Check sheet for the modelled part. Datum: model origin and axes. Units: mm. A direction names the side the tool comes from. Round coordinates to 2 decimals unless told otherwise and drop trailing zeros. Write each loop counter-clockwise with the first axis right and the second up, starting at its lowest first coordinate (ties: lowest second). Pieces come first, ordered by that corner, then holes.
from build123d import *

# Parameters (mm, degrees)
BOSS_EXTRU_1_DEPTH      = 18.275
ESQUISSE2_W             = 40
ESQUISSE2_H             = 22
BOSS_EXTRU_2_DEPTH      = 3
ESQUISSE3_W             = 40
ESQUISSE3_H             = 2
BOSS_EXTRU_3_DEPTH      = 2
ESQUISSE4_W             = 20
ESQUISSE4_H             = 2
ENL_V_MAT_EXTRU_2_DEPTH = 22.275
ENL_V_START             = -7.775
ESQUISSE5_W             = 31.2
ESQUISSE5_H             = 5
ENL_V_MAT_EXTRU_3_DEPTH = 7.775
ESQUISSE6_W             = 34
ESQUISSE6_H             = 5.725
ENL_V_MAT_EXTRU_4_DEPTH = 12.5
BOSS_EXTRU_4_DEPTH      = 21.275
ESQUISSE8_W             = 34
ESQUISSE8_H             = 5.725
ENL_V_MAT_EXTRU_5_DEPTH = 11.946457824


with BuildPart() as part:
    # Esquisse1 → Boss.-Extru.1 (new body)
    with BuildSketch(Plane.XY):
        Polygon((-15.6, -80), (-20, -80), (-20, -60), (20, -60), (20, -80), (15.6, -80), (15.6, -76.5), (8.8, -76.5), (8.8, -71.5), (-8.8, -71.5), (-8.8, -76.5), (-15.6, -76.5), align=None)
    extrude(amount=BOSS_EXTRU_1_DEPTH)

    # Esquisse2 → Boss.-Extru.2 (add)
    with BuildSketch(Plane.XY.offset(18.275)):
        with Locations((0, -71)):
            Rectangle(ESQUISSE2_W, ESQUISSE2_H)
    extrude(amount=BOSS_EXTRU_2_DEPTH)

    # Esquisse3 → Boss.-Extru.3 (add)
    with BuildSketch(Plane(origin=(0, 0, 18.275), x_dir=(-1, 0, 0), z_dir=(0, 0, -1))):
        with Locations((0, -81)):
            Rectangle(ESQUISSE3_W, ESQUISSE3_H)
    extrude(amount=BOSS_EXTRU_3_DEPTH)

    # Esquisse4 → Enlèv. mat.-Extru.2 (cut, through all)
    with BuildSketch(Plane.XY.offset(21.275)):
        with Locations((0, -81)):
            Rectangle(ESQUISSE4_W, ESQUISSE4_H)
    extrude(amount=-ENL_V_MAT_EXTRU_2_DEPTH, mode=Mode.SUBTRACT)

    # Esquisse5 → Enlèv. mat.-Extru.3 (cut)
    with BuildSketch(Plane(origin=(0, 0, 0), x_dir=(-1, 0, 0), z_dir=(0, 0, -1)).offset(ENL_V_START)):
        with Locations((0, -74)):
            Rectangle(ESQUISSE5_W, ESQUISSE5_H)
    extrude(amount=ENL_V_MAT_EXTRU_3_DEPTH, mode=Mode.SUBTRACT)

    # Esquisse6 → Enlèv. mat.-Extru.4 (cut, through all)
    with BuildSketch(Plane.XZ.offset(71.5)):
        with Locations((0, 2.8625)):
            Rectangle(ESQUISSE6_W, ESQUISSE6_H)
    extrude(amount=-ENL_V_MAT_EXTRU_4_DEPTH, mode=Mode.SUBTRACT)

    # Esquisse7 → Boss.-Extru.4 (add)
    with BuildSketch(Plane.XY.offset(21.275)):
        with BuildLine():
            Line((-30, -49.053542176), (-20, -82))
            Line((-20, -82), (-18, -82))
            Line((-18, -82), (-18, -60))
            Line((-18, -60), (18, -60))
            Line((18, -60), (18, -82))
            Line((18, -82), (20, -82))
            Line((20, -82), (30, -49.053542176))
            ThreePointArc((30, -49.053542176), (0, -57.5), (-30, -49.053542176))
        make_face()
    extrude(amount=-BOSS_EXTRU_4_DEPTH)

    # Esquisse8 → Enlèv. mat.-Extru.5 (cut, through all)
    with BuildSketch(Plane.XZ.offset(60)):
        with Locations((0, 2.8625)):
            Rectangle(ESQUISSE8_W, ESQUISSE8_H)
    extrude(amount=-ENL_V_MAT_EXTRU_5_DEPTH, mode=Mode.SUBTRACT)


solid = part.part
1. Sectioned sample at D-D, the plane y = -65. Enter the section's corners in (x, z) (3 decimals), plus the area to 3 significant figures.
2. Sectioned sample at B-B, the plane z = 11.25. Enter the section's corners in (x, y), plus the area to 3 significant figures.
3. Go/stop test with flat-tipped pins: pin 1 (9.5 mm diameter, centred on y = -77, z = 5.5, fed in from -X); pin 2 (1.6 mm diameter, centred on x = 13.5, z = 17.5, fed in from +Y); pin 3 (0.7 mm diameter, centred on x = 16.5, z = 1.5, fed in from +Y). Record where each tip stops, or that it passes through.
4. Sectioned sample at C-C, the plane y = -53.5. Enter the section's corners in (x, z) (3 decimals), plus the area to 3 significant figures.
5. Sectioned sample at A-A, the plane z = 2.25. Enter the section's corners in (x, y), plus the area to 3 significant figures.
6. Release check for a two-part mould opening along X. For faces 1 (the cylindrical face through (0.4, -57.5, 10.8)), 2 (the flat face through (-21, -65, 0)), 3 (the flat face through (18, -81, 8)), 4 (the flat face through (24.93, -65.76, 10.79)) record: released by +X, released by -X, zero draft, split by the parting line, or undercut.
7. Set-up check for faces 5 (the flat face through (-25.07, -65.3, 10.79)), 6 (the flat face through (21, -65, 0)), 7 (the flat face through (10, -81, 19)), 8 (the flat face through (-13, -80, 17)), 9 (the flat face through (-18, -81, 8)): record each of +Z, -Z, +X, -X, +Y, -Y from which the full face is reachable in a straight line by a thin tool's end or side.
8. Scan lines: line 1 along X through (y, z) = (-77, 15.75); line 2 along Z through (x, y) = (12, -61) (3 decimals); line 3 along X through (y, z) = (-59, 5.5). Record each from-to range of solid material in increasing order.
Computed values:
1. outline: (-25.16, 0) - (-17, 0) - (-17, 5.725) - (17, 5.725) - (17, 0) - (25.16, 0) - (25.16, 21.275) - (-25.16, 21.275) - close
1. area: 876 mm2
2. outline: (-30, -49.05) - (-20, -82) - (-18, -82) - (-18, -80) - (-15.6, -80) - (-15.6, -76.5) - (-8.8, -76.5) - (-8.8, -71.5) - (8.8, -71.5) - (8.8, -76.5) - (15.6, -76.5) - (15.6, -80) - (18, -80) - (18, -82) - (20, -82) - (30, -49.05) arc R57.5 cw to start
2. area: 1,030 mm2
3. pin 1: stops at x = -22.96
3. pin 2: stops at y = -55.69
3. pin 3: stops at y = -71.5
4. outline: (-28.65, 0) - (-21.071, 0) - (-21.071, 21.275) - (-28.65, 21.275) - close; (21.071, 0) - (28.65, 0) - (28.65, 21.275) - (21.071, 21.275) - close
4. area: 322 mm2
5. outline: (-30, -49.05) - (-20, -82) - (-18, -82) - (-18, -80) - (-15.6, -80) - (-15.6, -71.5) - (-17, -71.5) - (-17, -54.93) arc R57.5 cw to start; (15.6, -80) - (18, -80) - (18, -82) - (20, -82) - (30, -49.05) arc R57.5 cw to (17, -54.93) - (17, -71.5) - (15.6, -71.5) - close
5. area: 462 mm2
6. face 1: undercut
6. face 2: zero draft
6. face 3: undercut
6. face 4: released by +X
7. face 5: +Z, -Z, -X, -Y
7. face 6: -Z, +X, -X, +Y, -Y
7. face 7: +Z, -Z, -Y
7. face 8: -Z
7. face 9: -Z, -Y
8. line 1: x = -21.52 to -15.6, 15.6 to 21.52
8. line 2: z = 5.725 to 21.275
8. line 3: x = -26.98 to -17, 17 to 26.98
